from build123d import *

# Parameters (mm, degrees)
SKETCH_1_W      = 70
SKETCH_1_H      = 70
SKETCH_1_R      = 15
EXTRUDE_1_DEPTH = 10
SCALE_1_SCALE   = 0.6


with BuildPart() as part:
    # 草图1 → 凸台-拉伸1 (new body)
    with BuildSketch(Plane.XY):
        Rectangle(SKETCH_1_W, SKETCH_1_H)
        Circle(SKETCH_1_R, mode=Mode.SUBTRACT)
    extrude(amount=EXTRUDE_1_DEPTH)


with BuildPart() as part_1:
    # 缩放比例1: scaled about (0, 0, 0)
    add(part.part.scale(SCALE_1_SCALE))


solid = part_1.part
For this review, take the finished solid that the model builds, in its own axes (mm). Round coordinates to 2 decimals unless told otherwise and drop trailing zeros. Loops run counter-clockwise (first coordinate to the right, second up) from the corner with the lowest first, then second, coordinate; pieces in that order, holes last. Notation, with made-up numbers: (-29, -6) - (-20, -6) arc R18 cw to (-20, -2) - close; hole circle Ø6 at (23, 88.25). An arc over 180 degrees is marked (long way). One line per question, with ' | ' between items.
Q1. For pin 1 (8 mm diameter, centred on x = 2, y = -4.5, fed in from +Z); pin 2 (10 mm diameter, centred on x = -1, y = -14.5, fed in from -Z), all flat-tipped, find the tip position at first contact; note any pin that passes through.
Taken from the geometry:
pin 1: passes through | pin 2: stops at z = 0
Q2. Take a section at C-C (z = 3.65). Give the boundary of the cut face in (x, y), and give its area (3 significant figures).
Taken from the geometry:
outline: (-21, -21) - (21, -21) - (21, 21) - (-21, 21) - close; hole circle Ø18 at (0, 0) | area: 1,510 mm²
Q3. The part is to be moulded in two halves that separate along X. For faces 1 (the flat face through (21, 0, 3)), 2 (the flat face through (-10, 0, 0)), 3 (the cylindrical face through (-1.172, 8.923, 2.958)), 4 (the flat face through (-21, 0, 3)), say which applies: released by +X, released by -X, zero draft, split by the parting line, or undercut.
Taken from the geometry:
face 1: released by +X | face 2: zero draft | face 3: undercut | face 4: released by -X
Q4. Take a section at A-A (x = 0). Give the boundary of the cut face in (y, z), and give its area (3 significant figures).
Taken from the geometry:
outline: (-21, 0) - (-9, 0) - (-9, 6) - (-21, 6) - close; (9, 0) - (21, 0) - (21, 6) - (9, 6) - close | area: 144 mm²
Q5. For line 1 along Y through (x, z) = (0, 4.05); line 2 along Y through (x, z) = (7, 1.95); line 3 along X through (y, z) = (6.5, 3.8), list the stretches that pass through material, from the lowest coordinate up. Write a range as [from, to].
Taken from the geometry:
line 1: y = [-21, -9], [9, 21] | line 2: y = [-21, -5.66], [5.66, 21] | line 3: x = [-21, -6.22], [6.22, 21]
